CAD build for the part. Positions are in the model's coordinates, mm. Give positions to 0.01 mm unless a question says otherwise; leave off trailing zeros. Write each loop counter-clockwise with the first axis right and the second up, starting at its lowest first coordinate (ties: lowest second). Pieces come first, ordered by that corner, then holes. Notation, with made-up numbers: (-4, -23) -> (37, -23) arc R13 ccw to (37, 2) -> close; hole circle Ø8 at (14, -7). An arc over 180 degrees is marked (long way). Answer as a JSON object with one key per item and string values.
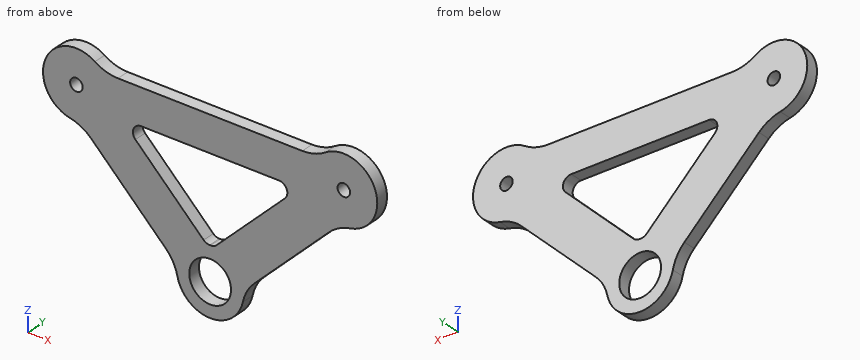
```python
from build123d import *

# Parameters (mm, degrees)
SKETCH2_R           = 1.5
SKETCH2_R_2         = 5
BOSS_EXTRUDE1_DEPTH = 3
FILLET1_R           = 10
FILLET2_R           = 2


with BuildPart() as part:
    # Sketch2 → Boss-Extrude1 (new body)
    with BuildSketch(Plane(origin=(0, 0, 0), x_dir=(1, 0, 0), z_dir=(0, 1, 0))):
        with BuildLine():
            Line((-25.755002002, -7.091520556), (25.755002002, -7.091520556))
            ThreePointArc((25.755002002, -7.091520556), (39.399896119, -5.131510265), (31.07348397, 5.854646321))
            Line((31.07348397, 5.854646321), (7.956268299, 28.711722383))
            ThreePointArc((7.956268299, 28.711722383), (8.3294e-05, 37.547063483), (-7.956285692, 28.711888061))
            Line((-7.956285692, 28.711888061), (-31.074510761, 5.854765977))
            ThreePointArc((-31.074510761, 5.854765977), (-39.399699694, -5.131988356), (-25.755002002, -7.091520556))
        make_face()
        with Locations(Location((-32, -2.091520556, 0), (0, 0, 270))):
            Circle(SKETCH2_R, mode=Mode.SUBTRACT)
        with Locations(Location((32, -2.091520556, 0), (0, 0, 270))):
            Circle(SKETCH2_R, mode=Mode.SUBTRACT)
        with BuildLine():
            Line((0.92651603, 21.600896605), (21.348745942, 1.408479444))
            Line((21.348745942, 1.408479444), (-21.34844873, 1.408479444))
            Line((-21.34844873, 1.408479444), (-0.925489239, 21.60077695))
            ThreePointArc((-0.925489239, 21.60077695), (0.00051687, 21.5470635), (0.92651603, 21.600896605))
        make_face(mode=Mode.SUBTRACT)
        Polygon((0, 22.515813483), (0, 22.516986487), (0.000593189, 22.516399973), align=None, mode=Mode.SUBTRACT)
        with Locations(Location((0, 29.547063483, 0), (0, 0, 270))):
            Circle(SKETCH2_R_2, mode=Mode.SUBTRACT)
    extrude(amount=BOSS_EXTRUDE1_DEPTH)

    # Fillet1
    fillet1_edges = [part.edges().sort_by_distance(p)[0] for p in [
        (-25.755002002, 1.5, 7.091520556),
        (-31.074510761, 1.5, -5.854765977),
        (-7.956285692, 1.5, -28.711888061),
        (7.956268299, 1.5, -28.711722383),
        (31.07348397, 1.5, -5.854646321),
        (25.755002002, 1.5, 7.091520556),
    ]]
    fillet(fillet1_edges, radius=FILLET1_R)

    # Fillet2
    fillet2_edges = [part.edges().sort_by_distance(p)[0] for p in [
        (0.92651603, 1.5, -21.600896605),
        (-0.925489239, 1.5, -21.60077695),
        (-21.34844873, 1.5, -1.408479444),
        (21.348745942, 1.5, -1.408479444),
    ]]
    fillet(fillet2_edges, radius=FILLET2_R)


solid = part.part
```
1) Slice it at A-A (x = 32). List the corners of the cut face in (y, z).
Model answer:
{"outline": "(0, -6.19) -> (3, -6.19) -> (3, 0.59) -> (0, 0.59) -> close; (0, 3.59) -> (3, 3.59) -> (3, 10.09) -> (0, 10.09) -> close"}
2) Wall check: probe 1 along X at (y, z) = (1, -13); probe 2 along Z at (x, y) = (14, 2.8); probe 3 along Z at (x, y) = (6.5, 1.4). Give the ranges that are in metal, low to high.
Model answer:
{"probe 1": "x = -23.85 to -9.62, 9.63 to 23.85", "probe 2": "z = -22.74 to -8.67, -1.41 to 7.09", "probe 3": "z = -34.21 to -16.09, -1.41 to 7.09"}
3) Slice it at C-C (z = -4). List the corners of the cut face in (x, y).
Model answer:
{"outline": "(-37.19, 0) -> (-18.39, 0) -> (-18.39, 3) -> (-37.19, 3) -> close; (18.39, 0) -> (37.19, 0) -> (37.19, 3) -> (18.39, 3) -> close"}
4) Slice it at B-B (x = 4). List the corners of the cut face in (y, z), then the cut area to 3 significant figures.
Model answer:
{"outline": "(0, -36.48) -> (3, -36.48) -> (3, -32.55) -> (0, -32.55) -> close; (0, -26.55) -> (3, -26.55) -> (3, -18.56) -> (0, -18.56) -> close; (0, -1.41) -> (3, -1.41) -> (3, 7.09) -> (0, 7.09) -> close", "area": "61.2 mm2"}
5) Pin check, flat tips, straight feed: pin 1 (16 mm diameter, centred on x = 0, z = -29.55, fed in from +Y); pin 2 (1.5 mm diameter, centred on y = 2, z = -32, fed in from +X); pin 3 (1 mm diameter, centred on x = 24, y = 1.5, fed in from +Z). Stop position of each tip, or through.
Model answer:
{"pin 1": "stops at y = 3", "pin 2": "stops at x = 7.82", "pin 3": "stops at z = 7.4"}
